Work out the finished part from the listing and answer in its coordinate system (mm). Face numbers are marked on the shaded views. A direction names the side the tool comes from. Round coordinates to 2 decimals unless told otherwise and drop trailing zeros. Loops run counter-clockwise (first coordinate to the right, second up) from the corner with the lowest first, then second, coordinate; pieces in that order, holes last. Notation, with made-up numbers: (34.5, 0.25) - (85.5, 0.25) arc R19 cw to (85.5, 29.25) - close; hole circle Ø3 at (70, 63.5). An arc over 180 degrees is marked (long way). Answer as CSV lines item,"result". Start each with the question number.
Q1. Straight lines are drawn through the part: L1, parallel to X at y = 8, z = -24; L2, parallel to Y at x = 38, z = 0.5; L3, parallel to Y at x = 133, z = -3.5. For each, find the intervals that lie inside material, in ascending order. Write a range as [from, to].
Q2. Section C-C on x = 98 is taken. Write down the section's boundary in (y, z).
Q3. For the marked faces 4 and 5, determine the directions among +Z, -Z, +X, -X, +Y, -Y from which every point of the face is accessible in a straight line to the end or side of a thin tool.
Q4. Each of these flat-tipped pins is pushed along its axis until it touches: pin 1 Ø5 at (y, z) = (15.91, 15.91) entering from -X; pin 2 Ø12 at (x, z) = (27.5, 13.5) entering from +Y; pin 3 Ø3.5 at (y, z) = (-15.91, 15.91) entering from -X. Where does it stop, or does it pass through?
Q5. Section A-A on z = 0 is taken. Write down the section's boundary in (x, y), then the cut area to 3 significant figures.
Q6. Section D-D on y = -10.5 is taken. Write down the section's boundary in (x, z).
Q7. The mould has two halves that part along X. Classify the marked faces 1, 2 and 3: +X half, -X half, draft (parallel to the pull), parting line (faces both ways), or undercut.
```python
from build123d import *

# Parameters (mm, degrees)
SKETCH2_R          = 2.1
CUT_EXTRUDE1_DEPTH = 6.5


with BuildPart() as part:
    # Sketch1 → Revolve1 (revolve)
    with BuildSketch(Plane.XY):
        Polygon((0, 0), (153, 0), (153, 28.5), (128, 28.5), (128, 28), (93, 28), (93, 28.5), (78, 28.5), (78, 28), (28, 28), (28, 16), (26, 16), (26, 6), (0, 6), align=None)
    revolve(axis=Axis((-903.237381769, 0, 0), (1, 0, 0)))

    # Sketch2 → Cut-Extrude1 (cut)
    with BuildSketch(Plane.ZY.offset(-28)):
        with Locations((-15.909902577, 15.909902577)):
            Circle(SKETCH2_R)
        with Locations((15.909902577, 15.909902577)):
            Circle(SKETCH2_R)
        with Locations((15.909902577, -15.909902577)):
            Circle(SKETCH2_R)
        with Locations((-15.909902577, -15.909902577)):
            Circle(SKETCH2_R)
    extrude(amount=-CUT_EXTRUDE1_DEPTH, mode=Mode.SUBTRACT)


solid = part.part
```
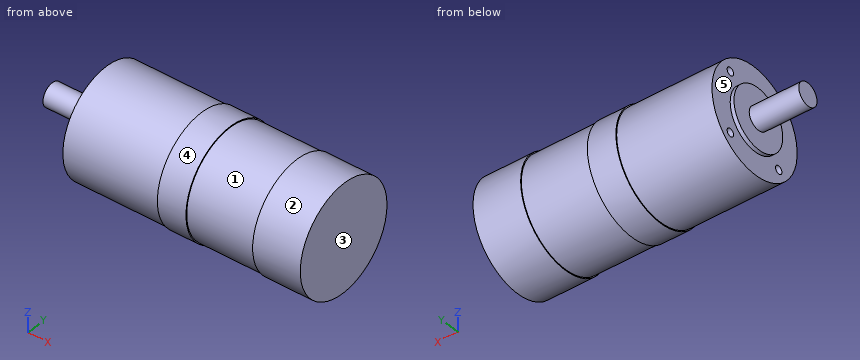
Findings:
1,L1,"x = [28, 153]"
1,L2,"y = [-28, 28]"
1,L3,"y = [-28.28, 28.28]"
2,outline,"circle Ø56 at (0, 0)"
3,face 4,"+X, -X"
3,face 5,"-X"
4,pin 1,"stops at x = 28"
4,pin 2,"stops at y = 26.97"
4,pin 3,"stops at x = 34.5"
5,outline,"(0, -6) - (26, -6) - (26, -16) - (28, -16) - (28, -28) - (78, -28) - (78, -28.5) - (93, -28.5) - (93, -28) - (128, -28) - (128, -28.5) - (153, -28.5) - (153, 28.5) - (128, 28.5) - (128, 28) - (93, 28) - (93, 28.5) - (78, 28.5) - (78, 28) - (28, 28) - (28, 16) - (26, 16) - (26, 6) - (0, 6) - close"
5,area,"7,420 mm^2"
6,outline,"(26, -12.07) - (28, -12.07) - (28, -25.96) - (78, -25.96) - (78, -26.5) - (93, -26.5) - (93, -25.96) - (128, -25.96) - (128, -26.5) - (153, -26.5) - (153, 26.5) - (128, 26.5) - (128, 25.96) - (93, 25.96) - (93, 26.5) - (78, 26.5) - (78, 25.96) - (28, 25.96) - (28, 12.07) - (26, 12.07) - close"
7,face 1,"undercut"
7,face 2,"draft"
7,face 3,"+X half"
